The drawing under review shows one solid part. Ordinate dimensions are in mm from its lowest x, y, z. A direction names the side the tool comes from. Coordinates: 2 decimals unless noted, no trailing zeros. Order: outer loops, then holes, each group sorted by start corner. A loop starts at its lowest first (then second) coordinate and runs counter-clockwise, first axis right, second up. Notation, with made-up numbers: (15, 39) -> (66, 39) arc R22 ccw to (66, 49) -> close; hole circle Ø4 at (78.5, 81.5). An arc over 180 degrees is marked (long way). Write item = value, one per line.
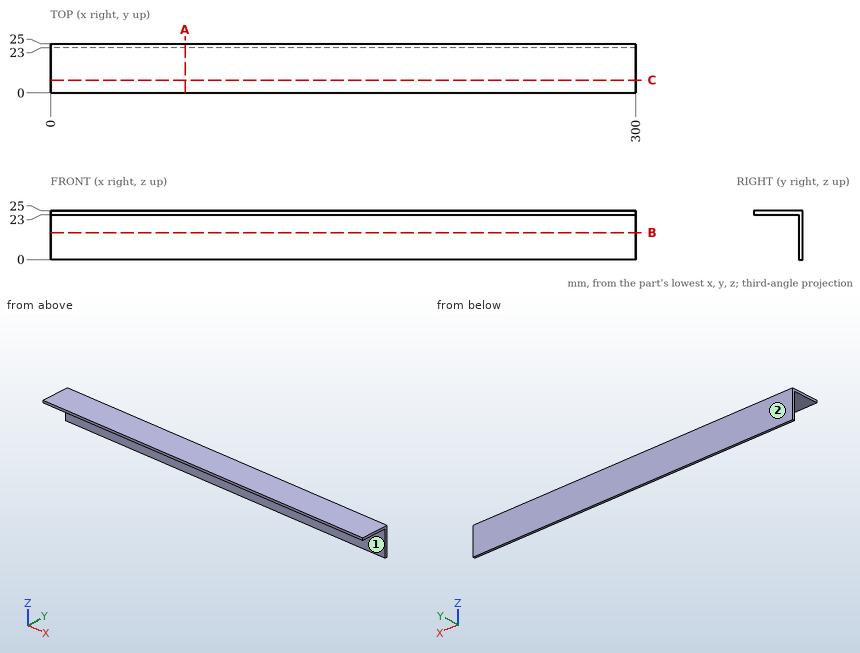
(1) For the marked faces 1 and 2, list the 3-axis set-ups (+Z, -Z, +X, -X, +Y, -Y) from which the entire face can be reached by the end or side of a thin tool; tool diameter is ignored.
Report:
face_1 = -Z, +X, -X, -Y
face_2 = +Z, -Z, +X, -X, +Y
(2) Insertion check: pin 1 (1.5 mm diameter, centred on y = 20.5, z = 21, fed in from +X); pin 2 (4 mm diameter, centred on x = 70.5, y = 20.5, fed in from -Z); pin 3 (3 mm diameter, centred on x = 266, z = 15.5, fed in from -Y). Each pin has a flat end and moves straight along its axis. Give the tip position at first contact, or say it passes through.
Report:
pin_1 = through
pin_2 = 23
pin_3 = 23
(3) We need section A-A (x = 69). Write out the cut boundary in (y, z), and give its area (3 significant figures).
Report:
outline = (0, 23) -> (23, 23) -> (23, 0) -> (25, 0) -> (25, 25) -> (0, 25) -> close
area = 96.0 mm²
(4) For L1, parallel to Y at x = 249, z = 5.25, list the stretches that pass through material, from the lowest coordinate up.
Report:
L1 = 23 to 25
(5) We need section B-B (z = 13.75). Write out the cut boundary in (x, y).
Report:
outline = (0, 23) -> (300, 23) -> (300, 25) -> (0, 25) -> close
